```python
from build123d import *

# Parameters (mm, degrees)
F0_W      = 8
F0_H      = 6
F1_DEPTH  = 8
F2_W      = 3.85
F2_H      = 3.85
F3_DEPTH  = 3
F4_W      = 8
F4_H      = 8
F4_W_2    = 3.85
F4_H_2    = 3.85
F5_DEPTH  = 2
F7_W      = 3.85
F7_H      = 3.85
F8_DEPTH  = 3
F9_W      = 8
F9_H      = 8
F9_W_2    = 3.85
F9_H_2    = 3.85
F10_DEPTH = 2.35
F11_DEPTH = 0.35
F12_DEPTH = 1
F13_DEPTH = 0.65
F14_DEPTH = 1


with BuildPart() as f1:
    # F0 (on Top) → F1 (new body)
    with BuildSketch(Plane.XY):
        Rectangle(F0_W, F0_H)
    extrude(amount=F1_DEPTH)

    # F2 (on face) → F3 (join)
    with BuildSketch(Plane.XZ.offset(3)):
        with Locations((0, 4)):
            Rectangle(F2_W, F2_H)
    extrude(amount=F3_DEPTH)

    # F4 (on face) → F5 (join)
    with BuildSketch(Plane.XZ.offset(6)):
        with Locations((0, 4)):
            Rectangle(F4_W, F4_H)
        with Locations((0, 4)):
            Rectangle(F4_W_2, F4_H_2, mode=Mode.SUBTRACT)
        with Locations((0, 4)):
            Rectangle(F4_W_2, F4_H_2)
    extrude(amount=F5_DEPTH)

    # F7 (on face) → F8 (join)
    with BuildSketch(Plane(origin=(0, 3, 0), x_dir=(-1, 0, 0), z_dir=(0, 1, 0))):
        with Locations((0, 4)):
            Rectangle(F7_W, F7_H)
    extrude(amount=F8_DEPTH)

    # F9 (on face) → F10 (join)
    with BuildSketch(Plane(origin=(0, 6, 0), x_dir=(-1, 0, 0), z_dir=(0, 1, 0))):
        with Locations((0, 4)):
            Rectangle(F9_W, F9_H)
        with Locations((0, 4)):
            Rectangle(F9_W_2, F9_H_2, mode=Mode.SUBTRACT)
        with Locations((0, 4)):
            Rectangle(F9_W_2, F9_H_2)
    extrude(amount=F10_DEPTH)

    # F11 (add): a face of the model
    f11_faces = [f1.faces().sort_by_distance(p)[0] for p in [
        (-3.886862915, 6, 4),
    ]]
    extrude(f11_faces, amount=-F11_DEPTH)

    # F12 (cut): a face of the model
    f12_faces = [f1.faces().sort_by_distance(p)[0] for p in [
        (-3.886862915, 6, 4),
    ]]
    extrude(f12_faces, amount=-F12_DEPTH, mode=Mode.SUBTRACT)

    # F13 (add): a face of the model
    f13_faces = [f1.faces().sort_by_distance(p)[0] for p in [
        (0, 8.35, 4),
    ]]
    extrude(f13_faces, amount=F13_DEPTH)

    # F14 (add): a face of the model
    f14_faces = [f1.faces().sort_by_distance(p)[0] for p in [
        (0, 9, 4),
    ]]
    extrude(f14_faces, amount=F14_DEPTH)


solid = f1.part
```
Model file for the job. Use its own axes, mm. A direction names the side the tool comes from. Coordinates: 2 decimals unless noted, no trailing zeros. Order: outer loops, then holes, each group sorted by start corner. A loop starts at its lowest first (then second) coordinate and runs counter-clockwise, first axis right, second up. Notation, with made-up numbers: (-35.75, 9.25) -> (-11.75, 9.25) arc R19 ccw to (-11.75, 25.25) -> close; hole circle Ø10 at (-28, 75.5). An arc over 180 degrees is marked (long way). Answer as a JSON object with one key per item and string values. Group by question number.
1) Pull direction Y, two halves, no side cores. Call faces 6 (the face through (0, -8, 4)), 7 (the face through (1.925, 5, 4)), 8 (the face through (0, 10, 4)): +Y half, -Y half, draft (parallel to the pull), parting line (faces both ways), or undercut.
2) Cut at D-D, the plane z = 5.25. Write the cut outline in (x, y) (3 decimals), then the cut area to 3 significant figures.
3) Drill centre lines: L1, parallel to Y at x = -2.5, z = 3; L2, parallel to Z at x = -1.75, y = 5.75 (3 decimals); L3, parallel to X at y = 3.5, z = 4.5 (3 decimals). Where is each one in solid material? Low to high.
4) Cut at C-C, the plane x = 1. Write the cut outline in (y, z) (3 decimals), then the cut area to 3 significant figures.
5) Flat gauge pins, fed straight in: pin 1 (1.5 mm diameter, centred on x = 0, y = -4, fed in from +Z) (3 decimals); pin 2 (1.5 mm diameter, centred on x = 0, y = -4, fed in from -Z) (3 decimals); pin 3 (0.9 mm diameter, centred on y = -5, z = 3.5, fed in from +X) (3 decimals). Where does each tip first touch, or does it go through?
6) Cut at A-A, the plane z = 1.75. Write the cut outline in (x, y), then the cut area to 3 significant figures.
7) Which spindle directions (+Z, -Z, +X, -X, +Y, -Y) get a long thin tool onto all of the face, cutting with end or side? Do faces 1 (the face through (-1.925, -4, 4)), 2 (the face through (1.925, -4, 4)), 3 (the face through (0, 7, 1)), 4 (the face through (0, 5, 5.925)), 5 (the face through (0, -7, 0)). Say none if no direction does.
8) Cut at B-B, the plane x = 3.25. Write the cut outline in (y, z), then the cut area to 3 significant figures.
Check values:
{
 "1": {"face 6": "-Y half", "face 7": "undercut", "face 8": "+Y half"},
 "2": {"outline": "(-4, -8) -> (4, -8) -> (4, -6) -> (1.925, -6) -> (1.925, -3) -> (4, -3) -> (4, 3) -> (1.925, 3) -> (1.925, 7) -> (4, 7) -> (4, 10) -> (-4, 10) -> (-4, 7) -> (-1.925, 7) -> (-1.925, 3) -> (-4, 3) -> (-4, -3) -> (-1.925, -3) -> (-1.925, -6) -> (-4, -6) -> close", "area": "115 mm²"},
 "3": {"L1": "y = -8 to -6, -3 to 3, 7 to 10", "L2": "z = 2.075 to 5.925", "L3": "x = -1.925 to 1.925"},
 "4": {"outline": "(-8, 0) -> (-6, 0) -> (-6, 2.075) -> (-3, 2.075) -> (-3, 0) -> (3, 0) -> (3, 2.075) -> (7, 2.075) -> (7, 0) -> (10, 0) -> (10, 8) -> (7, 8) -> (7, 5.925) -> (3, 5.925) -> (3, 8) -> (-3, 8) -> (-3, 5.925) -> (-6, 5.925) -> (-6, 8) -> (-8, 8) -> close", "area": "115 mm²"},
 "5": {"pin 1": "stops at z = 5.925", "pin 2": "stops at z = 2.075", "pin 3": "stops at x = 1.925"},
 "6": {"outline": "(-4, -8) -> (4, -8) -> (4, -6) -> (-4, -6) -> close; (-4, -3) -> (4, -3) -> (4, 3) -> (-4, 3) -> close; (-4, 7) -> (4, 7) -> (4, 10) -> (-4, 10) -> close", "area": "88.0 mm²"},
 "7": {"face 1": "+Z, -Z, -X", "face 2": "+Z, -Z, +X", "face 3": "none", "face 4": "+Z, +X, -X", "face 5": "-Z, +X, -X, +Y, -Y"},
 "8": {"outline": "(-8, 0) -> (-6, 0) -> (-6, 8) -> (-8, 8) -> close; (-3, 0) -> (3, 0) -> (3, 8) -> (-3, 8) -> close; (7, 0) -> (10, 0) -> (10, 8) -> (7, 8) -> close", "area": "88.0 mm²"}
}
